Design review of the part built by this model. Coordinates are the model's own, in mm. A direction names the side the tool comes from. Give positions to 0.01 mm unless a question says otherwise; leave off trailing zeros. Write each loop counter-clockwise with the first axis right and the second up, starting at its lowest first coordinate (ties: lowest second). Pieces come first, ordered by that corner, then holes. Notation, with made-up numbers: M -19,54.25 L 14,54.25 A24 ccw 14,88.25 Z; hole C 81.25,-38 d10. An arc over 180 degrees is marked long. One line per item, written item: value. Start each with the question number.
```python
from build123d import *

# Parameters (mm, degrees)
SKETCH1_R             = 12.7
EXTRUDE1_DEPTH        = 50.8
SHELL1_T              = -3.175
F_4_40_TAPPED_HOLE1_D = 2.2606
F_4_40_TAPPED_HOLE2_D = 2.2606
SKETCH8_R             = 3.571875
CUT_EXTRUDE1_DEPTH    = 54.881536726


with BuildPart() as part:
    # Sketch1 → Extrude1 (new body)
    with BuildSketch(Plane(origin=(0, 0, 0), x_dir=(1, 0, 0), z_dir=(0, 1, 0))):
        with Locations(Location((0, 0, 0), (0, 0, 270))):
            Circle(SKETCH1_R)
    extrude(amount=EXTRUDE1_DEPTH)

    # Shell1
    shell1_openings = [part.faces().sort_by_distance(p)[0] for p in [
        (0, 50.8, 0),
    ]]
    offset(amount=SHELL1_T, openings=shell1_openings, kind=Kind.INTERSECTION)

    # #4-40 Tapped Hole1 (through all)
    with Locations(Plane(origin=(0, 0, 7.14375), x_dir=(0, 0, -1), z_dir=(0, -1, 0))):
        with Locations((0, 0)):
            Hole(F_4_40_TAPPED_HOLE1_D / 2)

    # #4-40 Tapped Hole2 (through all)
    with Locations(Plane(origin=(0, 0, -7.14375), x_dir=(0, 0, -1), z_dir=(0, -1, 0))):
        with Locations((0, 0)):
            Hole(F_4_40_TAPPED_HOLE2_D / 2)

    # Sketch8 → Cut-Extrude1 (cut, through all)
    with BuildSketch(Plane.XZ):
        with Locations(Location((0, 0, 0), (0, 0, 270))):
            Circle(SKETCH8_R)
    extrude(amount=-CUT_EXTRUDE1_DEPTH, mode=Mode.SUBTRACT)


solid = part.part
```
Q1. Wall thickness on line 1 (X direction, y = 31, z = 0) (3 decimals); line 2 (Z direction, x = -0.25, y = 39.5); line 3 (X direction, y = 1.2, z = 0): over which ranges is each line inside the solid? List them lowest first. Write a range as from..to.
Q2. Take a section at B-B, the plane x = 0. Give the boundary of the cut face in (y, z) (3 decimals).
Q3. Take a section at A-A, the plane z = 0. Give the boundary of the cut face in (x, y) (3 decimals), then the cut area to 3 significant figures.
Q4. Machinability: for faces 1 (the face through (0.05, 1.61, -8.273)), 2 (the face through (-5.796, 26.654, -7.559)), which of the approach directions +Z, -Z, +X, -X, +Y, -Y give a long, thin tool a straight path to every point of the face, cutting with its end or side? Answer none if there is none.
Q5. Take a section at C-C, the plane x = -3. Give the boundary of the cut face in (y, z) (3 decimals).
Q6. For P1, Ø4, axis at y = 15, z = 6, coming from the -X side; P2, Ø1.5, axis at x = 2.5, y = 29.5, coming from the -Z side; P3, Ø5, axis at x = -7.5, y = 29.5, coming from the -Z side, all flat-tipped, find the tip position at first contact; note any pin that passes through.
Q7. The part is to be moulded in two halves that separate along X. For faces 3 (the face through (-0.4, 1.6, 8.2)), 4 (the face through (-7.7, 25, -10.1)), 5 (the face through (-3, 0, 3)), say which applies: pulls with the +X half, pulls with the -X half, needs draft (parallel to the pull), parting line crosses it, or undercut.
Q8. Take a section at D-D, the plane y = 34. Give the boundary of the cut face in (x, z) (3 decimals), then the cut area to 3 significant figures.
Results list:
1. line 1: x = -12.7..-9.525, 9.525..12.7
1. line 2: z = -12.7..-9.52, 9.52..12.7
1. line 3: x = -12.7..-3.57, 3.57..12.7
2. outline: M 0,-12.7 L 50.8,-12.7 L 50.8,-9.525 L 3.175,-9.525 L 3.175,-8.274 L 0,-8.274 Z; M 0,-6.013 L 3.175,-6.013 L 3.175,-3.572 L 0,-3.572 Z; M 0,3.572 L 3.175,3.572 L 3.175,6.013 L 0,6.013 Z; M 0,8.274 L 3.175,8.274 L 3.175,9.525 L 50.8,9.525 L 50.8,12.7 L 0,12.7 Z
3. outline: M -12.7,0 L -3.572,0 L -3.572,3.175 L -9.525,3.175 L -9.525,50.8 L -12.7,50.8 Z; M 3.572,0 L 12.7,0 L 12.7,50.8 L 9.525,50.8 L 9.525,3.175 L 3.572,3.175 Z
3. area: 360 mm^2
4. face 1: +Y, -Y
4. face 2: +Y
5. outline: M 0,-12.341 L 50.8,-12.341 L 50.8,-9.04 L 3.175,-9.04 L 3.175,-1.939 L 0,-1.939 Z; M 0,1.939 L 3.175,1.939 L 3.175,9.04 L 50.8,9.04 L 50.8,12.341 L 0,12.341 Z
6. P1: stops at x = -12.05
6. P2: stops at z = -12.58
6. P3: stops at z = -11.67
7. face 3: undercut
7. face 4: parting line crosses it
7. face 5: needs draft
8. outline: C 0,0 d25.4; hole C 0,0 d19.05
8. area: 222 mm^2
